```python
from build123d import *

# Parameters (mm, degrees)
SKETCH1_W                 = 83
SKETCH1_H                 = 100
BOSS_EXTRUDE1_DEPTH       = 1.5875
BOSS_EXTRUDE2_DEPTH       = 0.25
F_0_CLEARANCE_HOLE1_D     = 1.778
F_0_CLEARANCE_HOLE1_DEPTH = 3.175
F_0_CLEARANCE_HOLE1_TIP   = 0.53416509


with BuildPart() as part:
    # Sketch1 → Boss-Extrude1 (new body)
    with BuildSketch(Plane.XY):
        Rectangle(SKETCH1_W, SKETCH1_H)
    extrude(amount=BOSS_EXTRUDE1_DEPTH)

    # Sketch2 → Boss-Extrude2 (add)
    with BuildSketch(Plane.XY.offset(1.5875)):
        Polygon((-36.5, 45), (36.5, 45), (39, 42.5), (39, 30.5), (36.5, 28), (-36.5, 28), (-39, 30.5), (-39, 42.5), align=None)
        Polygon((-36.5, 26.75), (36.5, 26.75), (39, 24.25), (39, 12.25), (36.5, 9.75), (-36.5, 9.75), (-39, 12.25), (-39, 24.25), align=None)
        Polygon((-36.5, 8.5), (36.5, 8.5), (39, 6), (39, -6), (36.5, -8.5), (-36.5, -8.5), (-39, -6), (-39, 6), align=None)
        Polygon((-36.5, -9.75), (36.5, -9.75), (39, -12.25), (39, -24.25), (36.5, -26.75), (-36.5, -26.75), (-39, -24.25), (-39, -12.25), align=None)
        Polygon((-36.5, -28), (36.5, -28), (39, -30.5), (39, -42.5), (36.5, -45), (-36.5, -45), (-39, -42.5), (-39, -30.5), align=None)
    extrude(amount=BOSS_EXTRUDE2_DEPTH)

    # #0 Clearance Hole1
    with Locations(Plane.XY.offset(1.5875)):
        with Locations((-39, 45), (-39, 27), (-39, 9), (-39, -9), (-39, -27), (-39, -45), (39, -45), (39, -27), (39, -9), (39, 9), (39, 27), (39, 45)):
            Hole(F_0_CLEARANCE_HOLE1_D / 2, depth=F_0_CLEARANCE_HOLE1_DEPTH)
            with Locations((0, 0, -(F_0_CLEARANCE_HOLE1_DEPTH + F_0_CLEARANCE_HOLE1_TIP / 2))):  # 118° drill point
                Cone(0, F_0_CLEARANCE_HOLE1_D / 2, F_0_CLEARANCE_HOLE1_TIP, mode=Mode.SUBTRACT)


solid = part.part
```
Geometry check sheet. Reference: the model listing, model coordinates, mm. Round coordinates to 2 decimals unless told otherwise and drop trailing zeros. Order: outer loops, then holes, each group sorted by start corner. A loop starts at its lowest first (then second) coordinate and runs counter-clockwise, first axis right, second up. Notation, with made-up numbers: (45, 32.5) - (102, 32.5) arc R17 ccw to (102, 44.5) - close; hole circle Ø2 at (43, -27.75). An arc over 180 degrees is marked (long way). Use a Markdown table: item, result. Add a question column.
1) Section check A-A (x = 0.5). Record the cut outline in (y, z).
2) Gauge pin test, flat end, axial feed: P1, Ø1.1, axis at x = -39, y = 45, coming from the -Z side. Record the tip position at first contact, or that the pin passes through.
3) Thickness scan on line 1 along X through (y, z) = (45, 0.3); line 2 along Y through (x, z) = (5, 1.7); line 3 along X through (y, z) = (-9.5, 1.35). Record the ranges inside material, lowest first.
Established:
| question | item | result |
|---|---|---|
| 1 | outline | (-50, 0) - (50, 0) - (50, 1.59) - (45, 1.59) - (45, 1.84) - (28, 1.84) - (28, 1.59) - (26.75, 1.59) - (26.75, 1.84) - (9.75, 1.84) - (9.75, 1.59) - (8.5, 1.59) - (8.5, 1.84) - (-8.5, 1.84) - (-8.5, 1.59) - (-9.75, 1.59) - (-9.75, 1.84) - (-26.75, 1.84) - (-26.75, 1.59) - (-28, 1.59) - (-28, 1.84) - (-45, 1.84) - (-45, 1.59) - (-50, 1.59) - close |
| 2 | P1 | through |
| 3 | line 1 | -41.5 to -39.89, -38.11 to 38.11, 39.89 to 41.5 |
| 3 | line 2 | -45 to -28, -26.75 to -9.75, -8.5 to 8.5, 9.75 to 26.75, 28 to 45 |
| 3 | line 3 | -41.5 to -39.74, -38.26 to 38.26, 39.74 to 41.5 |
